Could you check a few things on this model? Use its own coordinates, in mm. A direction names the side the tool comes from. Give positions to 0.01 mm unless a question says otherwise; leave off trailing zeros. Order: outer loops, then holes, each group sorted by start corner. A loop starts at its lowest first (then second) coordinate and runs counter-clockwise, first axis right, second up. Notation, with made-up numbers: (28, 61.25) -> (75, 61.25) arc R37 cw to (75, 97.25) -> close; hole circle Ø9 at (-31, -28.75). An arc over 180 degrees is marked (long way). Answer as CSV lines item,"result". Start each with the question number.
(1) Will these pins go through, and if not, where does the flat tip stop? pin 1 Ø1.5 at (x, z) = (2.5, 37) entering from +Y; pin 2 Ø1.8 at (y, z) = (-60, 57) entering from +X; pin 3 Ø8 at (x, z) = (3, 8.5) entering from -Y.
(2) I want a section at C-C (x = 11). Please give me the cut outline in (y, z).
(3) I want a section at A-A (y = -39). Please give me the cut outline in (x, z).
(4) I want a section at D-D (y = -23). Please give me the cut outline in (x, z).
(5) On a 3-axis mill with a long thin cutter (end or side, diameter ignored), from which of +Z, -Z, +X, -X, +Y, -Y can I reach the whole of each face in a straight line? I mean faces 1 (the face through (0.14, -11.3, 28.25)), 2 (the face through (-5.5, -85, 31)), 3 (the face through (-5.5, -60, 56)), 4 (the face through (-9.74, -68.23, 48.8)), 5 (the face through (0, -35, 17)). Say none if no direction works.
(6) We'd pull the mould along Z, two halves only. Please class faces 6 (the face through (6.25, -25, 12)), 7 (the face through (0.22, -64.16, 10.19)), 8 (the face through (-0.22, -77.51, 35.01)), 9 (the face through (0.14, -38.8, 28.25)): released by +Z, released by -Z, zero draft, split by the parting line, or undercut.
(7) I need wall thicknesses on L1, parallel to Z at x = 6, y = -26.5; L2, parallel to Z at x = -7, y = -39; L3, parallel to Y at x = 0, z = 26.5. Which ranges of each line are inside material? Lowest first, please.
(8) I want a section at B-B (z = 21). Please give me the cut outline in (x, y), plus the area to 3 significant figures.
```python
from build123d import *

# Parameters (mm, degrees)
F1_DEPTH  = 32
F2_R      = 32
F3_DEPTH  = 19
F4_R      = 9.5
F5_DEPTH  = 19
F6_R      = 19.5
F6_R_2    = 9.5
F7_DEPTH  = 12
F9_DEPTH  = 11
F10_R     = 10
F12_DEPTH = 12.5
F13_R     = 12.5
F14_DEPTH = 15
F15_R     = 12.5
F16_DEPTH = 15
F17_R     = 7.5
F18_DEPTH = 70
F20_D     = 10
F21_SCALE = 0.5


with BuildPart() as f1:
    # F0 (on Right) → F1 (new body, symmetric)
    with BuildSketch(Plane.YZ):
        Polygon((-140, 0), (0, 0), (0, 19), (-129.0303448854, 19), (-159.0455173281, 70.9878036687), (-131.332704407, 86.9878036687), (-140.832704407, 103.4422863406), (-185, 77.9422863406), align=None)
    extrude(amount=F1_DEPTH, both=True)

    # F2 (on face) → F3 (join, through all)
    with BuildSketch(Plane(origin=(0, -80, 138.5640646055), x_dir=(1, 0, 0), z_dir=(0, -0.5, 0.8660254038))):
        with Locations((0, -70.2435565298)):
            Circle(F2_R)
    extrude(amount=-F3_DEPTH)

    # F4 (on face) → F5 (cut, through all)
    with BuildSketch(Plane(origin=(0, -80, 138.5640646055), x_dir=(1, 0, 0), z_dir=(0, -0.5, 0.8660254038))):
        with Locations((0, -70.2435565298)):
            Circle(F4_R)
    extrude(amount=-F5_DEPTH, mode=Mode.SUBTRACT)

    # F6 (on face) → F7 (cut)
    with BuildSketch(Plane(origin=(0, -80, 138.5640646055), x_dir=(1, 0, 0), z_dir=(0, -0.5, 0.8660254038))):
        with Locations((0, -70.2435565298)):
            Circle(F6_R)
        with Locations((0, -70.2435565298)):
            Circle(F6_R_2, mode=Mode.SUBTRACT)
    extrude(amount=-F7_DEPTH, mode=Mode.SUBTRACT)

    # F8 (on Right) → F9 (cut, symmetric)
    with BuildSketch(Plane.YZ):
        Polygon((-176.8038475773, 75.7461339179), (-102.4204401346, 118.6914142282), (-139.8535072803, 145.4511135817), (-219.7459042072, 72.3169818521), (-158.4675441277, 28.5975767315), (-151.8038475773, 32.4448637287), align=None)
    extrude(amount=F9_DEPTH, both=True, mode=Mode.SUBTRACT)

    # F10
    f10_edges = [f1.edges().sort_by_distance(p)[0] for p in [
        (0, -159.045517, 70.987804),
        (0, -129.030345, 19),
    ]]
    fillet(f10_edges, radius=F10_R)

    # F11 (on Right) → F12 (join, symmetric)
    with BuildSketch(Plane.YZ):
        Polygon((-85, 44), (-85, 19), (-15, 19), (-15, 44), (-30, 44), (-30, 26), (-70, 26), (-70, 44), align=None)
    extrude(amount=F12_DEPTH, both=True)

    # F13 (on face) → F14 (join, through all)
    with BuildSketch(Plane.XZ.offset(85)):
        with Locations((0, 44)):
            Circle(F13_R)
    extrude(amount=-F14_DEPTH)

    # F15 (on face) → F16 (join, through all)
    with BuildSketch(Plane.XZ.offset(30)):
        with Locations((0, 44)):
            Circle(F15_R)
    extrude(amount=-F16_DEPTH)

    # F17 (on face) → F18 (cut, through all)
    with BuildSketch(Plane(origin=(0, -15, 0), x_dir=(-1, 0, 0), z_dir=(0, 1, 0))):
        with Locations((0, 44)):
            Circle(F17_R)
    extrude(amount=-F18_DEPTH, mode=Mode.SUBTRACT)

    # F20 (through all)
    with Locations(Plane.YZ.offset(32)):
        with Locations((-97.6659357548, 9.6274418756)):
            Hole(F20_D / 2)


with BuildPart() as f1_1:
    # F21: moved
    add(f1.part.scale(F21_SCALE))


solid = f1_1.part
```
Final values:
1,pin 1,"y = -75.57"
1,pin 2,"x = 11.84"
1,pin 3,"y = -77.22"
2,outline,"(-92.5, 38.97) -> (-70, 0) -> (0, 0) -> (0, 9.5) -> (-61.63, 9.5) arc R5 cw to (-65.96, 12) -> (-77.02, 31.16) arc R5 cw to (-75.19, 37.99) -> (-55.6, 49.3) -> (-60.35, 57.53) -> close; hole circle Ø5 at (-48.83, 4.81)"
3,outline,"(-16, 0) -> (16, 0) -> (16, 9.5) -> (6.25, 9.5) -> (6.25, 22) arc R6.25 ccw to (-6.25, 22) -> (-6.25, 9.5) -> (-16, 9.5) -> close; hole circle Ø7.5 at (0, 22)"
4,outline,"(-16, 0) -> (16, 0) -> (16, 9.5) -> (6.25, 9.5) -> (6.25, 13) -> (-6.25, 13) -> (-6.25, 9.5) -> (-16, 9.5) -> close"
5,face 1,"+Z, +Y"
5,face 2,"-Y"
5,face 3,"+Z, -Y"
5,face 4,"none"
5,face 5,"+Z, +X, -X"
6,face 6,"zero draft"
6,face 7,"undercut"
6,face 8,"undercut"
6,face 9,"released by +Z"
7,L1,"0 to 13"
7,L2,"0 to 9.5"
7,L3,"-81.84 to -74.33, -42.5 to -35, -15 to -7.5"
8,outline,"(-16, -82.12) -> (-5.5, -82.12) -> (-5.5, -78.66) -> (5.5, -78.66) -> (5.5, -82.12) -> (16, -82.12) -> (16, -71.15) -> (-16, -71.15) -> close; (-6.25, -42.5) -> (-3.61, -42.5) -> (-3.61, -35) -> (-6.25, -35) -> close; (-6.25, -15) -> (-3.61, -15) -> (-3.61, -7.5) -> (-6.25, -7.5) -> close; (3.61, -42.5) -> (6.25, -42.5) -> (6.25, -35) -> (3.61, -35) -> close; (3.61, -15) -> (6.25, -15) -> (6.25, -7.5) -> (3.61, -7.5) -> close"
8,area,"392 mm²"
